```python
from build123d import *

# Parameters (mm, degrees)
BOSS_EXTRUDE1_START     = -109.652
BOSS_EXTRUDE1_DEPTH     = 9.525
CUT_EXTRUDE1_DEPTH      = 1399.485644649
CUT_EXTRUDE1_DEPTH_BACK = 1399.485644649
CUT_EXTRUDE2_START      = -103.127
CUT_EXTRUDE2_DEPTH      = 1296.358644649


with BuildPart() as part:
    # Sketch1 → Boss-Extrude1 (new body)
    with BuildSketch(Plane(origin=(0, 0, 0), x_dir=(0, 0, -1), z_dir=(1, 0, 0)).offset(BOSS_EXTRUDE1_START)):
        Polygon((-1044.923144897, 473.87249639), (-1311.176339914, 430.114447736), (-1297.268878193, 345.492161514), (-1031.015683176, 389.250210169), align=None)
    extrude(amount=BOSS_EXTRUDE1_DEPTH)

    # Sketch2 → Cut-Extrude1 (cut, two sides: drawn at the far end of the back side and taken through both)
    with BuildSketch(Plane(origin=(0, 0, 0), x_dir=(0, 0, -1), z_dir=(1, 0, 0)).offset(-CUT_EXTRUDE1_DEPTH_BACK)):
        with BuildLine():
            Line((-1108.923879409, 412.894172152), (-1115.653599818, 411.788159384))
            ThreePointArc((-1115.653599818, 411.788159384), (-1117.305228207, 410.762789477), (-1117.748059826, 408.869865828))
            Line((-1117.748059826, 408.869865828), (-1114.045674009, 386.34207761))
            ThreePointArc((-1114.045674009, 386.34207761), (-1113.020304102, 384.690449222), (-1111.127380454, 384.247617603))
            Line((-1111.127380454, 384.247617603), (-1104.397660044, 385.35363037))
            ThreePointArc((-1104.397660044, 385.35363037), (-1102.746031655, 386.379000278), (-1102.303200036, 388.271923926))
            Line((-1102.303200036, 388.271923926), (-1106.005585853, 410.799712144))
            ThreePointArc((-1106.005585853, 410.799712144), (-1107.03095576, 412.451340533), (-1108.923879409, 412.894172152))
        make_face()
        with BuildLine():
            Line((-1206.337571934, 371.174134332), (-1210.039957751, 393.70192255))
            ThreePointArc((-1210.039957751, 393.70192255), (-1209.597126132, 395.594846198), (-1207.945497743, 396.620216105))
            Line((-1207.945497743, 396.620216105), (-1201.215777333, 397.726228873))
            ThreePointArc((-1201.215777333, 397.726228873), (-1199.322853685, 397.283397254), (-1198.297483778, 395.631768865))
            Line((-1198.297483778, 395.631768865), (-1194.595097961, 373.103980647))
            ThreePointArc((-1194.595097961, 373.103980647), (-1195.03792958, 371.211056999), (-1196.689557968, 370.185687092))
            Line((-1196.689557968, 370.185687092), (-1203.419278378, 369.079674324))
            ThreePointArc((-1203.419278378, 369.079674324), (-1205.312202026, 369.522505943), (-1206.337571934, 371.174134332))
        make_face()
    extrude(amount=CUT_EXTRUDE1_DEPTH + CUT_EXTRUDE1_DEPTH_BACK, mode=Mode.SUBTRACT)

    # Sketch3 → Cut-Extrude2 (cut, through all)
    with BuildSketch(Plane(origin=(0, 0, 0), x_dir=(0, 0, -1), z_dir=(1, 0, 0)).offset(CUT_EXTRUDE2_START)):
        with BuildLine():
            Line((-1095.503116711, 383.770114016), (-1114.13319278, 380.708307472))
            ThreePointArc((-1114.13319278, 380.708307472), (-1115.623683889, 381.056993797), (-1116.431061795, 382.357488633))
            Line((-1116.431061795, 382.357488633), (-1122.416828748, 418.778892809))
            ThreePointArc((-1122.416828748, 418.778892809), (-1122.068142423, 420.269383918), (-1120.767647587, 421.076761824))
            Line((-1120.767647587, 421.076761824), (-1102.137571518, 424.138568369))
            ThreePointArc((-1102.137571518, 424.138568369), (-1100.647080409, 423.789882043), (-1099.839702503, 422.489387207))
            Line((-1099.839702503, 422.489387207), (-1093.85393555, 386.067983031))
            ThreePointArc((-1093.85393555, 386.067983031), (-1094.202621875, 384.577491922), (-1095.503116711, 383.770114016))
        make_face()
        with BuildLine():
            Line((-1194.429469443, 408.97062509), (-1213.059545512, 405.908818545))
            ThreePointArc((-1213.059545512, 405.908818545), (-1214.360040348, 405.10144064), (-1214.708726673, 403.61094953))
            Line((-1214.708726673, 403.61094953), (-1208.722959719, 367.189545354))
            ThreePointArc((-1208.722959719, 367.189545354), (-1207.915581814, 365.889050518), (-1206.425090705, 365.540364193))
            Line((-1206.425090705, 365.540364193), (-1187.795014635, 368.602170738))
            ThreePointArc((-1187.795014635, 368.602170738), (-1186.4945198, 369.409548643), (-1186.145833474, 370.900039753))
            Line((-1186.145833474, 370.900039753), (-1192.131600428, 407.321443929))
            ThreePointArc((-1192.131600428, 407.321443929), (-1192.938978333, 408.621938765), (-1194.429469443, 408.97062509))
        make_face()
    extrude(amount=-CUT_EXTRUDE2_DEPTH, mode=Mode.SUBTRACT)


solid = part.part
```
Here's how the part is built. I have some questions about the finished solid (model axes, mm). A direction names the side the tool comes from. Give positions to 0.01 mm unless a question says otherwise; leave off trailing zeros. Order: outer loops, then holes, each group sorted by start corner. A loop starts at its lowest first (then second) coordinate and runs counter-clockwise, first axis right, second up. Notation, with made-up numbers: (8, 31.5) - (53, 31.5) arc R17 cw to (53, 53.5) - close; hole circle Ø11 at (-8.5, -35.5). An arc over 180 degrees is marked (long way). Answer as a JSON object with one key per item and string values. Group by question number.
Item 1: If we section it at A-A on x = -105: Please give me the cut outline in (y, z).
Item 2: Please list where these lines run through material, in increasing order: probe 1 along Z at (x, y) = (-108, 397); probe 2 along Z at (x, y) = (-107, 401); probe 3 along Y at (x, z) = (-105, 1202.5).
Item 3: If we section it at B-B on z = 1138: Please give me the cut outline in (x, y).
Item 4: Which directions (+Z, -Z, +X, -X, +Y, -Y) give clear straight access to the entire face, cutting with the end or side of a thin tool? Please do faces 1 (the flat face through (-104.956, 430.969, 1037.872)), 2 (the flat face through (-103.127, 408, 1105)).
Item 5: For P1, Ø4, axis at x = -102, y = 411.5, coming from the -Z side; P2, Ø2, axis at x = -104.5, z = 1267, coming from the +Y side; P3, Ø14.5, axis at y = 410, z = 1110.5, coming from the -X side, each with a flat end and sliding along its axis, tell me the tip position at first contact or that it passes through.
Item 6: If we section it at C-C on y = 356: Please give me the cut outline in (x, z), and give its area (3 significant figures).
Result set:
{
 "1": {"outline": "(345.49, 1297.27) - (389.25, 1031.02) - (473.87, 1044.92) - (430.11, 1311.18) - close; hole (365.54, 1206.43) - (368.6, 1187.8) arc R2 ccw to (370.9, 1186.15) - (407.32, 1192.13) arc R2 ccw to (408.97, 1194.43) - (405.91, 1213.06) arc R2 ccw to (403.61, 1214.71) - (367.19, 1208.72) arc R2 ccw to start; hole (380.71, 1114.13) - (383.77, 1095.5) arc R2 ccw to (386.07, 1093.85) - (422.49, 1099.84) arc R2 ccw to (424.14, 1102.14) - (421.08, 1120.77) arc R2 ccw to (418.78, 1122.42) - (382.36, 1116.43) arc R2 ccw to start"},
 "2": {"probe 1": "1032.29 to 1095.65, 1118.84 to 1190.44, 1213.62 to 1305.73", "probe 2": "1032.95 to 1096.31, 1119.49 to 1191.09, 1214.28 to 1306.39", "probe 3": "361.07 to 366.19, 407.64 to 447.98"},
 "3": {"outline": "(-109.65, 371.67) - (-100.13, 371.67) - (-100.13, 458.58) - (-109.65, 458.58) - close"},
 "4": {"face 1": "-Z, +X, -X, +Y", "face 2": "-X"},
 "5": {"P1": "z = 1034.34", "P2": "y = 437.54", "P3": "x = -103.13"},
 "6": {"outline": "(-109.65, 1233.33) - (-100.13, 1233.33) - (-100.13, 1299) - (-109.65, 1299) - close", "area": "625 mm²"}
}
